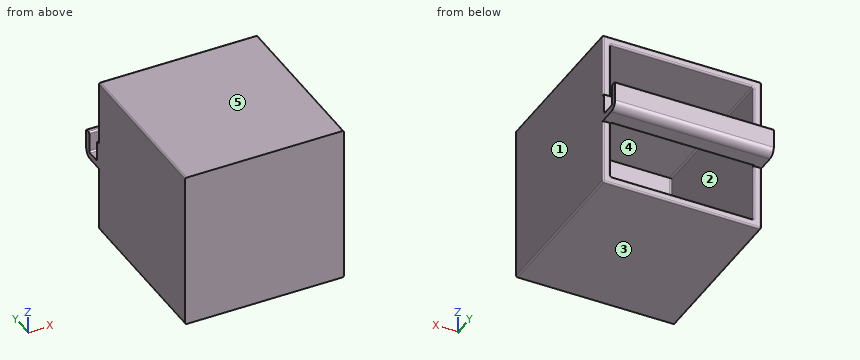
from build123d import *

# Parameters (mm, degrees)
SKETCH1_W               = 200
SKETCH1_H               = 200
SKETCH1_W_2             = 180
SKETCH1_H_2             = 180
BOSS_EXTRUDE1_DEPTH     = 200
SKETCH2_W               = 200
SKETCH2_H               = 200
BOSS_EXTRUDE2_DEPTH     = 10
SKETCH3_W               = 200
SKETCH3_H               = 35
BOSS_EXTRUDE3_DEPTH     = 30
CUT_EXTRUDE1_DEPTH      = 321.780298647
CUT_EXTRUDE1_DEPTH_BACK = 321.780298647
SKETCH4_W               = 26.954773083
SKETCH4_H               = 19
FILLET1_R               = 10
FILLET3_R               = 2
FILLET4_R               = 2
FILLET6_R               = 2
FILLET7_R               = 2
FILLET8_R               = 2
FILLET9_R               = 2


with BuildPart() as part:
    # Sketch1 → Boss-Extrude1 (new body)
    with BuildSketch(Plane(origin=(0, 0, 0), x_dir=(1, 0, 0), z_dir=(0, 1, 0))):
        Rectangle(SKETCH1_W, SKETCH1_H)
        Rectangle(SKETCH1_W_2, SKETCH1_H_2, mode=Mode.SUBTRACT)
    extrude(amount=BOSS_EXTRUDE1_DEPTH)

    # Sketch2 → Boss-Extrude2 (add)
    with BuildSketch(Plane.XZ):
        Rectangle(SKETCH2_W, SKETCH2_H)
    extrude(amount=BOSS_EXTRUDE2_DEPTH)

    # Sketch3 → Boss-Extrude3 (add)
    with BuildSketch(Plane(origin=(0, 200, 0), x_dir=(1, 0, 0), z_dir=(0, 1, 0))):
        Rectangle(SKETCH3_W, SKETCH3_H)
    extrude(amount=BOSS_EXTRUDE3_DEPTH)

    # Sketch4 → Cut-Extrude1 (cut, two sides: drawn at the far end of the back side and taken through both)
    with BuildSketch(Plane(origin=(100, 0, 0), x_dir=(0, 0, -1), z_dir=(1, 0, 0)).offset(-CUT_EXTRUDE1_DEPTH_BACK)):
        with Locations((-4.022613458, 212.997200487)):
            Rectangle(SKETCH4_W, SKETCH4_H)
    extrude(amount=CUT_EXTRUDE1_DEPTH + CUT_EXTRUDE1_DEPTH_BACK, mode=Mode.SUBTRACT)

    # Fillet1
    fillet1_edges = [part.edges().sort_by_distance(p)[0] for p in [
        (0, 230, -17.5),
    ]]
    fillet(fillet1_edges, radius=FILLET1_R)

    # Fillet3
    fillet3_edges = [part.edges().sort_by_distance(p)[0] for p in [
        (0, 200, -17.5),
    ]]
    fillet(fillet3_edges, radius=FILLET3_R)

    # Fillet4
    fillet4_edges = [part.edges().sort_by_distance(p)[0] for p in [
        (-100, 200, -58.75),
        (90, 0, 0),
        (90, 100, 90),
        (0, 0, -90),
        (90, 100, -90),
        (-90, 0, 0),
        (-90, 100, -90),
        (-90, 100, 90),
        (90, 200, 53.75),
        (0, 200, 100),
        (0, 200, -90),
        (-90, 200, -53.75),
        (0, 200, 90),
        (100, 200, -58.75),
        (-100, 200, 58.75),
        (90, 200, -53.75),
        (-90, 200, 53.75),
        (100, 200, 58.75),
        (100, 95, 100),
        (-100, 95, 100),
        (-100, 95, -100),
        (100, 95, -100),
        (0, 200, -100),
    ]]
    fillet(fillet4_edges, radius=FILLET4_R)

    # Fillet6
    fillet6_edges = [part.edges().sort_by_distance(p)[0] for p in [
        (0, 200, 17.5),
    ]]
    fillet(fillet6_edges, radius=FILLET6_R)

    # Fillet7
    fillet7_edges = [part.edges().sort_by_distance(p)[0] for p in [
        (0, 203.497200487, -9.454773083),
    ]]
    fillet(fillet7_edges, radius=FILLET7_R)

    # Fillet8
    fillet8_edges = [part.edges().sort_by_distance(p)[0] for p in [
        (0, 230, 17.5),
        (0, 222.497200487, -9.454773083),
        (0, 222.497200487, 17.5),
    ]]
    fillet(fillet8_edges, radius=FILLET8_R)

    # Fillet9
    # the kernel refuses this fillet: 2 mm, written as the material it takes off along each edge
    with BuildSketch(Plane(origin=(-105, 203.497200487, 17.5), x_dir=(0, 0, -1), z_dir=(1, 0, 0))) as fillet9_piece_1:
        with BuildLine():
            CenterArc((FILLET9_R, -FILLET9_R), FILLET9_R, 90, 90)
            Line((0, -FILLET9_R), (0, 0))
            Line((0, 0), (FILLET9_R, 0))
        make_face()
    extrude(amount=210, mode=Mode.SUBTRACT)


solid = part.part
The listing builds one solid part. Answer for the finished solid, in the listing's coordinates (mm). Face numbers are marked on the shaded views. A direction names the side the tool comes from. Give positions to 0.01 mm unless a question says otherwise; leave off trailing zeros. Write each loop counter-clockwise with the first axis right and the second up, starting at its lowest first coordinate (ties: lowest second). Pieces come first, ordered by that corner, then holes.
1) Find the intervals of material crossed by L1, parallel to Y at x = 13, z = 15; L2, parallel to X at y = 24, z = -51, in increasing order.
2) Section A-A (y = 186) is taken. Write down the section's boundary in (x, z).
3) For a pull along Z with two mould halves and no side action, classify the marked faces 1, 2 and 3 as pulls with the +Z half, pulls with the -Z half, needs draft (parallel to the pull), parting line crosses it, or undercut.
4) Section B-B (x = -71) is taken. Write down the section's boundary in (y, z), and give its area (3 significant figures).
5) Section C-C (z = 72.5) is taken. Write down the section's boundary in (x, y), and give its area (3 significant figures).
6) A tool of negligible diameter and unlimited length cuts with its end or side. For the marked faces 4 and 5, from which of +Z, -Z, +X, -X, +Y, -Y can it reach the whole face along a straight path? Write none if from no direction.
7) Given P1, Ø24, axis at x = 31, z = 49.5, coming from the +Y side; P2, Ø1.7, axis at x = 95, y = 199, coming from the +Z side; P3, Ø16.5, axis at x = 5, y = 216.5, coming from the +Z side, each flat-ended and moving along its own axis, determine where each tip first touches the part or whether it passes through.
Response:
1. L1: y = -10 to 0, 200 to 203.5, 222.5 to 230
1. L2: x = -100 to -90, 90 to 100
2. outline: (-100, -98) arc R2 ccw to (-98, -100) - (98, -100) arc R2 ccw to (100, -98) - (100, 98) arc R2 ccw to (98, 100) - (-98, 100) arc R2 ccw to (-100, 98) - close; hole (-90, -88) arc R2 ccw to (-88, -90) - (88, -90) arc R2 ccw to (90, -88) - (90, 88) arc R2 ccw to (88, 90) - (-88, 90) arc R2 ccw to (-90, 88) - close
3. face 1: needs draft
3. face 2: undercut
3. face 3: pulls with the -Z half
4. outline: (-10, -100) - (198, -100) arc R2 ccw to (200, -98) - (200, -92) arc R2 ccw to (198, -90) - (2, -90) arc R2 cw to (0, -88) - (0, 90) - (198, 90) arc R2 ccw to (200, 92) - (200, 98) arc R2 ccw to (198, 100) - (-10, 100) - close; (200, -15.5) arc R2 ccw to (202, -17.5) - (220, -17.5) arc R10 ccw to (230, -7.5) - (230, 15.5) arc R2 ccw to (228, 17.5) - (224.5, 17.5) arc R2 ccw to (222.5, 15.5) - (222.5, -7.45) arc R2 cw to (220.5, -9.45) - (205.5, -9.45) arc R2 cw to (203.5, -7.45) - (203.5, 15.5) arc R2 ccw to (201.75, 17.48) arc R2 ccw to (200, 15.5) - close
4. area: 6,510 mm2
5. outline: (-100, -10) - (100, -10) - (100, 198) arc R2 ccw to (98, 200) - (92, 200) arc R2 ccw to (90, 198) - (90, 2) arc R2 cw to (88, 0) - (-88, 0) arc R2 cw to (-90, 2) - (-90, 198) arc R2 ccw to (-92, 200) - (-98, 200) arc R2 ccw to (-100, 198) - close
5. area: 6,000 mm2
6. face 4: +Y
6. face 5: +Z, +X, -X, +Y, -Y
7. P1: stops at y = 0
7. P2: stops at z = 99.99
7. P3: stops at z = 17.5
